Autodesk Inventor part; units mm, degrees
ref_plane "YZ Plane" through (0, 0, 0) normal (1, 0, 0) x (0, 1, 0)
ref_plane "XZ Plane" through (0, 0, 0) normal (0, 1, 0) x (-1, 0, 0)
ref_plane "XY Plane" through (0, 0, 0) normal (0, 0, 1) x (1, 0, 0)
sketch "Sketch1" plane through (0, 0, 0) normal (1, 0, 0) x (0, 1, 0)
  line L0 (0, 0) -> (0, 10.6)
  line L1 (0, 10.6) -> (6, 10.6)
  line L2 (6, 0) -> (6, 9) construction
  line L3 (6, 10.6) -> (6, 9)
  line L4 (6, 9) -> (7.5, 9)
  line L5 (7.5, 9) -> (7.5, 11)
  line L6 (7.5, 11) -> (9.5, 11)
  line L7 (9.5, 11) -> (9.5, 12.5)
  line L8 (9.5, 11) -> (11, 11) construction
  line L9 (9.5, 12.5) -> (14.5, 12.5)
  line L10 (14.5, 0) -> (14.5, 10.5) construction
  line L11 (14.5, 12.5) -> (14.5, 10.5)
  line L12 (14.5, 10.5) -> (19.5, 10.5)
  line L13 (19.5, 0) -> (19.5, 9.2) construction
  line L14 (19.5, 10.5) -> (19.5, 9.2)
  line L15 (19.5, 9.2) -> (22.1, 9.2)
  line L16 (22.1, 9.2) -> (22.1, 10.5)
  line L17 (22.1, 10.5) -> (27.1, 10.5)
  line L18 (27.1, 10.5) -> (27.1, 0)
  line L19 (0, 0) -> (27.1, 0)
  dimension "d0" = 10.6
  dimension "d1" = 6
  dimension "d2" = 9
  dimension "d3" = 1.5
  dimension "d4" = 2
  dimension "d5" = 2
  dimension "d7" = 11
  dimension "d8" = 1.5
  dimension "d9" = 90
  dimension "d10" = 5
  dimension "d11" = 10.5
  dimension "d12" = 2
  dimension "d13" = 5
  dimension "d14" = 9.2
  dimension "d15" = 1.3
  dimension "d16" = 2.6
  dimension "d17" = 1.3
  dimension "d18" = 5
revolve "Revolution1" add sketch "Sketch1" angle 360 about axis through (0, 0, 0) along (0, 1, 0)
thread "Thread1"
chamfer "Chamfer1" distance 1 angle 45 1 edges at (0, 0, -10.6)
sketch "Sketch2" plane through (0, 27.1, 0) normal (0, 1, 0) x (1, 0, 0)
  circle A0 centre (0, 0) radius 7
  dimension "d25" = 14
extrude "Extrusion1" cut sketch "Sketch2" against normal through all
chamfer "Chamfer2" distance 1 angle 45 1 edges at (0, 27.1, -10.5)
sketch "Sketch3" plane through (0, 14.5, 0) normal (0, 1, 0) x (1, 0, 0)
  circle A0 centre (0, 0) radius 11
  circle A1 centre (0, 0) radius 11
  line L0 (0, 11) -> (-7.7224, 11)
  line L1 (-7.7224, 11) -> (-7.7224, 13.1204)
  line L2 (-7.7224, 13.1204) -> (0, 13.1204)
  line L3 (0, 13.1204) -> (0, 11)
  line L4 (0, 11) -> (7.8373, 11)
  line L5 (7.8373, 11) -> (7.8373, 13.1204)
  line L6 (7.8373, 13.1204) -> (0, 13.1204)
  line L7 (0, 13.1204) -> (0, 11)
  line L8 (0, -11) -> (-7.4786, -11)
  line L9 (-7.4786, -11) -> (-7.4786, -12.6458)
  line L10 (-7.4786, -12.6458) -> (0, -12.6458)
  line L11 (0, -12.6458) -> (0, -11)
  line L12 (0, -11) -> (7.7134, -11)
  line L13 (7.7134, -11) -> (7.7134, -12.6458)
  line L14 (7.7134, -12.6458) -> (0, -12.6458)
  line L15 (0, -12.6458) -> (0, -11)
  dimension "d31" = 22
extrude "Extrusion2" cut sketch "Sketch3" against normal through all contours L12 L13 L14 L11 | L11 L10 L9 L8 | L0 L1 L2 L3 | L3 L6 L5 L4
properties part number "Corrugated tube-Flowmeter connector" material "Polypropylene"
Check sheet for the modelled part. Datum: model origin and axes. Units: mm. A direction names the side the tool comes from. Round coordinates to 2 decimals unless told otherwise and drop trailing zeros. Order: outer loops, then holes, each group sorted by start corner. A loop starts at its lowest first (then second) coordinate and runs counter-clockwise, first axis right, second up. Notation, with made-up numbers: (-15, 58.25) - (31, 58.25) arc R13 cw to (31, 74.25) - close; hole circle Ø1 at (22, 66). An arc over 180 degrees is marked (long way). Write item = value, one per line.
Q1. Section check B-B (y = 20.75). Record the boundary of the cut face in (x, z), and give its area (3 significant figures).
Computed:
outline = circle Ø18.4 at (0, 0); hole circle Ø14 at (0, 0)
area = 112 mm^2
Q2. Go/stop test with a flat-tipped pin: pin 1 (1.5 mm diameter, centred on y = 22.5, z = -5.5, fed in from -X). Record where the tip stops, or that it passes through.
Computed:
pin_1 = -9.36
Q3. Section check A-A (y = 7). Record the boundary of the cut face in (x, z), and give its area (3 significant figures).
Computed:
outline = circle Ø18 at (0, 0); hole circle Ø14 at (0, 0)
area = 101 mm^2
Q4. Section check C-C (x = -10). State how many separate pieces and enclosed holes the cut face has, and give its area (3 significant figures).
Computed:
separate_pieces = 3
enclosed_holes = 0
area = 191 mm^2
Q5. Tool access check on faces 1 (the face through (0, 12, -11)), 2 (the face through (-8, 6, -5)), 3 (the face through (-4.06, 3.54, 9.79)), 4 (the face through (3.2, 24.1, 10)), 5 (the face through (11.4, 9.5, -0.1)). Record the directions out of +Z, -Z, +X, -X, +Y, -Y that give a thin tool (end or side, any length) a straight path to the whole face; none if there is none.
Computed:
face_1 = -Z, +X, -X, +Y, -Y
face_2 = none
face_3 = -Y
face_4 = +Y
face_5 = +X, -Y
Q6. Thickness scan on line 1 along Y through (x, z) = (4.75, 8); line 2 along X through (y, z) = (14.75, 0). Record the ranges inside material, lowest first.
Computed:
line_1 = 0 to 6, 7.5 to 19.5, 22.1 to 27.1
line_2 = -10.5 to -7, 7 to 10.5
Q7. Draft check along Y on faces 6 (the face through (-10.13, 14.5, -3.31)), 7 (the face through (12.5, 12, 0.2)), 8 (the face through (-7, 19.5, 6.2)), 9 (the face through (-11.3, 9.5, -0.1)). Enter one of: pulls with the +Y half, pulls with the -Y half, needs draft (parallel to the pull), parting line crosses it, or undercut.
Computed:
face_6 = pulls with the +Y half
face_7 = needs draft
face_8 = undercut
face_9 = pulls with the -Y half
